Here's how the part is built. I have some questions about the finished solid (model axes, mm). Face numbers are marked on the shaded views. Coordinates: 2 decimals unless noted, no trailing zeros. Write each loop counter-clockwise with the first axis right and the second up, starting at its lowest first coordinate (ties: lowest second). Pieces come first, ordered by that corner, then holes.
Item 1: I want a section at A-A (x = 0). Count the separate pieces of the cut face and the enclosed holes in it, and give its area (3 significant figures).
Item 2: If we mould it in two halves opening along X, with no side actions, what happens to the marked faces 1, 2 and 3? For each: pulls with the +X half, pulls with the -X half, needs draft (parallel to the pull), parting line crosses it, or undercut.
Item 3: Please list where these lines run through material, in increasing order: line 1 (Y direction, x = -19, z = 10.5); line 2 (Z direction, x = 7, y = 21.5); line 3 (X direction, y = 47, z = -4).
Item 4: I want a section at C-C (y = 19.5). Please give me the cut outline in (x, z), and give its area (3 significant figures).
Item 5: I want a section at B-B (z = 0). Please give me the cut outline in (x, y), and give its area (3 significant figures).
Item 6: I'm going to push flat-ended pins straight in: P1, Ø10, axis at x = 15, y = 11.5, coming from the +Z side; P2, Ø1, axis at x = -13, y = 17, coming from the -Z side; P3, Ø6, axis at x = 14.5, y = 55.5, coming from the +Z side. Where does each tip first touch, or does it pass through?
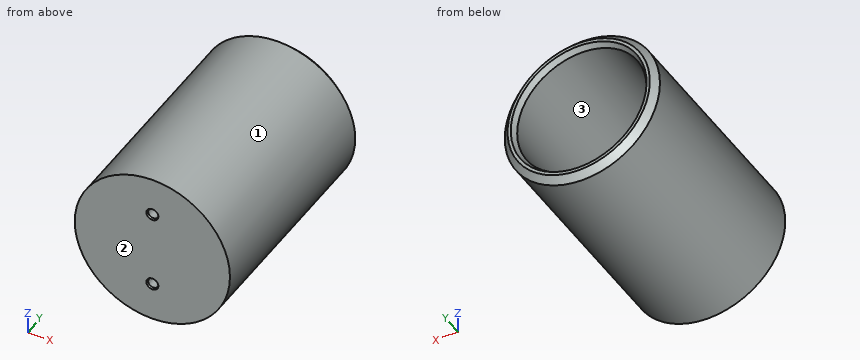
from build123d import *
from OCP.BRepFilletAPI import BRepFilletAPI_MakeChamfer

# Parameters (mm, degrees)
SKETCH2_R           = 30.48
BOSS_EXTRUDE2_DEPTH = 12.7
SKETCH3_R           = 4.125
CUT_EXTRUDE1_DEPTH  = 5.08
SKETCH4_R           = 2
CUT_EXTRUDE2_DEPTH  = 44.773567367
SKETCH5_R           = 30.48
SKETCH5_R_2         = 25.4
BOSS_EXTRUDE3_DEPTH = 76.2
CHAMFER1_SIZE       = 1.27
CHAMFER1_SIZE2      = 2.199704526
CHAMFER2_SIZE       = 2.54
CHAMFER3_SIZE       = 0.635
CHAMFER3_SIZE2      = 0.366617421


with BuildPart() as part:
    # Sketch2 → Boss-Extrude2 (new body)
    with BuildSketch(Plane(origin=(0, 0, 0), x_dir=(1, 0, 0), z_dir=(0, 1, 0))):
        with Locations(Location((0, 0, 0), (0, 0, 270))):
            Circle(SKETCH2_R)
    extrude(amount=BOSS_EXTRUDE2_DEPTH)

    # Sketch3 → Cut-Extrude1 (cut)
    with BuildSketch(Plane(origin=(0, 12.7, 0), x_dir=(1, 0, 0), z_dir=(0, 1, 0))):
        with Locations(Location((0, 15.24, 0), (0, 0, 270))):
            Circle(SKETCH3_R)
        with Locations(Location((0, -15.24, 0), (0, 0, 270))):
            Circle(SKETCH3_R)
    extrude(amount=-CUT_EXTRUDE1_DEPTH, mode=Mode.SUBTRACT)

    # Sketch4 → Cut-Extrude2 (cut, through all)
    with BuildSketch(Plane(origin=(0, 7.62, 0), x_dir=(1, 0, 0), z_dir=(0, 1, 0))):
        with Locations(Location((0, 15.24, 0), (0, 0, 270))):
            Circle(SKETCH4_R)
        with Locations(Location((0, -15.24, 0), (0, 0, 270))):
            Circle(SKETCH4_R)
    extrude(amount=-CUT_EXTRUDE2_DEPTH, mode=Mode.SUBTRACT)

    # Sketch5 → Boss-Extrude3 (add)
    with BuildSketch(Plane(origin=(0, 12.7, 0), x_dir=(1, 0, 0), z_dir=(0, 1, 0))):
        with Locations(Location((0, 0, 0), (0, 0, 270))):
            Circle(SKETCH5_R)
        with Locations(Location((0, 0, 0), (0, 0, 90))):
            Circle(SKETCH5_R_2, mode=Mode.SUBTRACT)
    extrude(amount=BOSS_EXTRUDE3_DEPTH)

    # Chamfer1
    chamfer1_edges = [part.edges().sort_by_distance(p)[0] for p in [
        (0, 88.9, 25.4),
    ]]
    chamfer1_side = [part.faces().sort_by_distance(p)[0] for p in [
        (0, 88.9, -29.617895412),
    ]]
    chamfer(chamfer1_edges, length=CHAMFER1_SIZE, length2=CHAMFER1_SIZE2, reference=chamfer1_side[0])

    # Chamfer2
    chamfer2_edges = [part.edges().sort_by_distance(p)[0] for p in [
        (0, 88.9, -30.48),
    ]]
    chamfer(chamfer2_edges, length=CHAMFER2_SIZE)

    # Chamfer3: one chamfer whose edges measure the first distance from different faces: ONE call of the kernel's chamfer builder (chamfer() names one face for all edges)
    chamfer3_edges_1 = [part.edges().sort_by_distance(p)[0] for p in [
        (0, 0, -17.24),
    ]]
    chamfer3_side_1 = [part.faces().sort_by_distance(p)[0] for p in [
        (0, 3.81, -17.24),
    ]]
    chamfer3_edges_2 = [part.edges().sort_by_distance(p)[0] for p in [
        (0, 0, 13.24),
    ]]
    chamfer3_side_2 = [part.faces().sort_by_distance(p)[0] for p in [
        (0, 3.81, 13.24),
    ]]
    chamfer3 = BRepFilletAPI_MakeChamfer(part.part.solid().wrapped)
    for e in chamfer3_edges_1:
        chamfer3.Add(CHAMFER3_SIZE, CHAMFER3_SIZE2, e.wrapped, chamfer3_side_1[0].wrapped)  # the first distance lies on this face
    for e in chamfer3_edges_2:
        chamfer3.Add(CHAMFER3_SIZE, CHAMFER3_SIZE2, e.wrapped, chamfer3_side_2[0].wrapped)  # the first distance lies on this face
    add(Compound.cast(chamfer3.Shape()), mode=Mode.REPLACE)


solid = part.part
Answer:
1. separate pieces: 3
1. enclosed holes: 0
1. area: 1,390 mm2
2. face 1: parting line crosses it
2. face 2: needs draft
2. face 3: undercut
3. line 1: y = 0 to 12.7
3. line 2: z = -29.67 to -24.42, 24.42 to 29.67
3. line 3: x = -30.22 to -25.08, 25.08 to 30.22
4. outline: circle Ø60.96 at (0, 0); hole circle Ø50.8 at (0, 0)
4. area: 892 mm2
5. outline: (-30.48, 0) - (30.48, 0) - (30.48, 86.36) - (27.94, 88.9) - (26.67, 88.9) - (25.4, 86.7) - (25.4, 12.7) - (-25.4, 12.7) - (-25.4, 86.7) - (-26.67, 88.9) - (-27.94, 88.9) - (-30.48, 86.36) - close
5. area: 1,540 mm2
6. P1: stops at z = 28.79
6. P2: stops at z = -27.8
6. P3: stops at z = 28.23
